Design review of the part built by this model. Coordinates are the model's own, in mm. Face numbers are marked on the shaded views. A direction names the side the tool comes from. Give positions to 0.01 mm unless a question says otherwise; leave off trailing zeros. Order: outer loops, then holes, each group sorted by start corner. A loop starts at its lowest first (then second) coordinate and runs counter-clockwise, first axis right, second up. Notation, with made-up numbers: (86.5, 16) -> (113.5, 16) arc R24 cw to (113.5, 50) -> close; hole circle Ø7 at (19.5, -29). An arc over 180 degrees is marked (long way). Use a Markdown table: item, result. Add a question column.
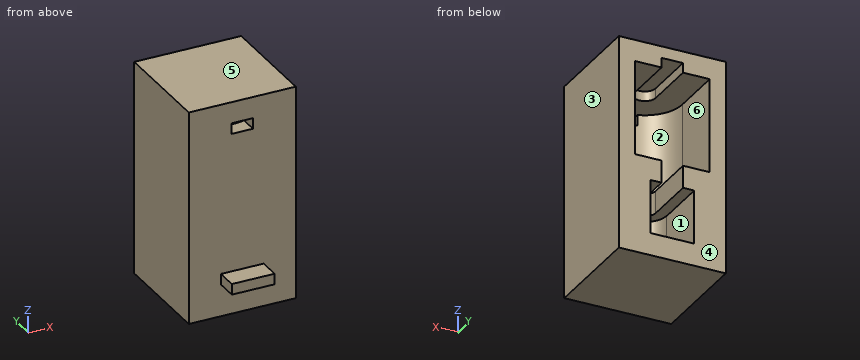
Autodesk Inventor part; units mm, degrees
ref_plane "Work Plane3" through (-14.75, 0, -89.55) normal (0, 0, -1) x (-1, 0, 0)
ref_plane "Work Plane4" through (-7.5, 0, -54) normal (0, 0, -1) x (-1, 0, 0)
ref_plane "Work Plane5" through (-14.75, 0, -64.45) normal (0, 0, -1) x (-1, 0, 0)
sketch "Sketch1" plane through (0, 0, 0) normal (0, 1, 0) x (-1, 0, 0)
  line L0 (0, 0) -> (50, 0)
  line L1 (50, 0) -> (50, -100)
  line L2 (50, -100) -> (0, -100)
  line L3 (0, -100) -> (0, 0)
  line L4 (25, 0) -> (25, -100)
  line L5 (7.5, -54) -> (7.5, -10)
  line L6 (7.5, -10) -> (42.5, -10)
  line L7 (42.5, -10) -> (42.5, -54)
  line L8 (42.5, -54) -> (7.5, -54)
  line L9 (7.5, -54) -> (42.5, -10) construction
  line L10 (7.5, -10) -> (42.5, -54) construction
  line L11 (7.5, -54) -> (51.5, -54) construction
  line L12 (14.75, -64.45) -> (14.75, -89.55)
  line L13 (14.75, -89.55) -> (35.25, -89.55)
  line L14 (35.25, -89.55) -> (35.25, -64.45)
  line L15 (35.25, -64.45) -> (14.75, -64.45)
  line L16 (14.75, -64.45) -> (35.25, -89.55) construction
  line L17 (14.75, -89.55) -> (35.25, -64.45) construction
  line L18 (14.75, -64.45) -> (39.85, -64.45) construction
  line L19 (25, -10) -> (25, -15)
  line L20 (25, -10) -> (30, -10) construction
  line L21 (20, -20) -> (30, -20)
  line L22 (30, -20) -> (30, -10)
  line L23 (30, -10) -> (20, -10)
  line L24 (20, -10) -> (20, -20)
  line L25 (20, -20) -> (30, -10) construction
  line L26 (30, -20) -> (20, -10) construction
  line L27 (20, -20) -> (30, -20) construction
  line L28 (30, -15) -> (20, -15)
  point P0 (25, -32)
  point P1 (25, -77)
  point P2 (25, -54)
  point P3 (25, -77)
  dimension "d0" = 50
  dimension "d1" = 100
  dimension "d4" = 44
  dimension "d5" = 90
  dimension "d6" = 35
  dimension "d7" = 10
  dimension "d8" = 25.1
  dimension "d9" = 90
  dimension "d10" = 20.5
  dimension "d35" = 5
  dimension "d36" = 90
  dimension "d37" = 0
extrude "Extrusion1" add sketch "Sketch1" against normal blind 50
ref_plane "Work Plane3" through (-14.75, 0, -89.55) normal (0, 0, -1) x (-1, 0, 0)
ref_plane "Work Plane4" through (-7.5, 0, -54) normal (0, 0, -1) x (-1, 0, 0)
sketch "Sketch3" plane through (-14.75, 0, -89.55) normal (0, 0, -1) x (-1, 0, 0)
  line L0 (35.25, 0) -> (-14.75, 0)
  line L1 (35.25, 0) -> (35.25, -50)
  line L2 (-14.75, -50) -> (35.25, -50)
  line L3 (-14.75, 0) -> (-14.75, -50)
  circle A0 centre (10.25, -25) radius 10.1
  line L4 (20.35, -35.1) -> (20.35, -14.9)
  line L5 (20.35, -14.9) -> (0.15, -14.9)
  line L6 (0.15, -14.9) -> (0.15, -35.1)
  line L7 (0.15, -35.1) -> (20.35, -35.1)
  line L8 (20.35, -35.1) -> (0.15, -14.9) construction
  line L9 (20.35, -14.9) -> (0.15, -35.1) construction
  line L10 (20.35, -35.1) -> (40.55, -35.1) construction
  point P0 (10.25, -35.1)
  point P1 (0.15, -25)
  point P2 (20.35, -25)
  dimension "d18" = 20.2
  dimension "d21" = 90
ref_plane "Work Plane5" through (-14.75, 0, -64.45) normal (0, 0, -1) x (-1, 0, 0)
ref_plane "Work Plane6" through (-7.5, 0, -10) normal (0, 0, -1) x (-1, 0, 0)
ref_plane "Work Plane7" through (-35.1, -35.1, -89.55) normal (0, 1, 0) x (1, 0, 0)
extrude "Extrusion5" cut sketch "Sketch1" against normal up to surface (35.1 mm away) contours L13 L12 L15 L4 | L4 L15 L14 L13
extrude "Extrusion6" add sketch "Sketch3" against normal up to surface (25.1 mm away) contours L4 L7 A0 | L7 L6 A0
sketch "Sketch4" plane through (-7.5, 0, -54) normal (0, 0, -1) x (-1, 0, 0)
  line L0 (42.5, 0) -> (-7.5, 0)
  line L1 (42.5, 0) -> (42.5, -50)
  line L2 (-7.5, -50) -> (42.5, -50)
  line L3 (-7.5, 0) -> (-7.5, -50)
  circle A0 centre (17.5, -25) radius 17.5
  line L4 (0, -42.5) -> (0, -7.5)
  line L5 (0, -7.5) -> (35, -7.5)
  line L6 (35, -7.5) -> (35, -42.5)
  line L7 (35, -42.5) -> (0, -42.5)
  line L8 (0, -42.5) -> (35, -7.5) construction
  line L9 (0, -7.5) -> (35, -42.5) construction
  line L10 (0, -42.5) -> (35, -42.5) construction
  point P0 (17.5, -42.5)
  point P1 (35, -25)
  point P2 (0, -25)
  dimension "d26" = 35
  dimension "d27" = 90
ref_plane "Work Plane8" through (-7.5, -42.5, -54) normal (0, 1, 0) x (1, 0, 0)
extrude "Extrusion7" cut sketch "Sketch1" against normal up to surface (42.5 mm away) contours L6 L22 L28 L4 | L4 L28 L24 L6 | L28 L22 L21 L4 | L4 L21 L24 L28 | L24 L21 L4 L8 L5 L6 | L6 L7 L8 L4 L21 L22
extrude "Extrusion8" add sketch "Sketch4" against normal up to surface (44 mm away) contours L6 L7 A0 | L7 L4 A0
sketch "Sketch5" plane through (-14.75, 0, -64.45) normal (0, 0, -1) x (-1, 0, 0)
  line L0 (35.25, 0) -> (-14.75, 0)
  line L1 (35.25, 0) -> (35.25, -50)
  line L2 (-14.75, -50) -> (35.25, -50)
  line L3 (-14.75, 0) -> (-14.75, -50)
  circle A0 centre (10.25, -25) radius 5
  dimension "d32" = 10
extrude "Extrusion9" cut sketch "Sketch5" against normal blind 59 contours A0
extrude "Extrusion10" cut sketch "Sketch1" against normal through all contours L6 L22 L28 L4 | L4 L28 L24 L6
ref_plane "Work Plane9" through (-25, -25, -64.45) normal (0, 1, 0) x (1, 0, 0)
sketch "Sketch6" plane through (-25, -25, -64.45) normal (0, 1, 0) x (1, 0, 0)
  line L0 (-5, 0) -> (-5, -10.45)
  line L1 (-5, 0) -> (5, 0)
  line L2 (5, -10.45) -> (-5, -10.45)
  line L3 (5, -10.45) -> (-5, -10.45)
  line L4 (-5, -10.45) -> (5, -10.45)
  line L5 (5, -10.45) -> (5, 0)
  line L6 (5, 0) -> (-5, 0)
  line L7 (-5, 0) -> (-5, -10.45)
  line L8 (-5, -59) -> (5, -59)
  line L9 (-5, -54.45) -> (-5, -59)
  line L10 (5, -54.45) -> (5, -59)
  line L11 (-5, -54.45) -> (5, -54.45)
  line L12 (5, -54.45) -> (-5, -54.45)
  line L13 (-5, -54.45) -> (-5, -59)
  line L14 (-5, -59) -> (5, -59)
  line L15 (5, -59) -> (5, -54.45)
  point P0 (25, -64.45)
extrude "Extrusion11" cut sketch "Sketch6" along normal through all
sketch "Sketch7" plane through (0, -50, 0) normal (0, -1, 0) x (1, 0, 0)
  line L0 (-50, -100) -> (0, -100)
  line L1 (-25, -100) -> (-25, -80)
  line L2 (-25, -80) -> (-35, -80)
  line L3 (-35, -80) -> (-35, -85)
  line L4 (-35, -85) -> (-25, -85)
  line L5 (-25, -85) -> (-25, -80)
  line L6 (-35, -85) -> (-15, -85)
  line L7 (-15, -85) -> (-15, -80)
  line L8 (-15, -80) -> (-35, -80)
  line L9 (-35, -80) -> (-35, -85)
  point P0 (0, 0)
  dimension "d42" = 20
  dimension "d43" = 10
  dimension "d44" = 5
  dimension "d45" = 20
extrude "Extrusion12" add sketch "Sketch7" along normal blind 10
properties part number "dcmotor_housing"
1) Add section A-A (x = -25). Give the boundary of the cut face in (y, z).
2) Add section D-D (y = -39). Give the boundary of the cut face in (x, z), then the cut area to 3 significant figures.
3) For L1, parallel to Z at x = -34.5, y = -7.5; L2, parallel to X at y = -5, z = -65; L3, parallel to Z at x = -34, y = -38, list the stretches that pass through material, from the lowest coordinate up. Write a range as [from, to].
4) Insertion check: pin 1 (10 mm diameter, centred on x = -20, z = -21.5, fed in from +Y); pin 2 (2 mm diameter, centred on x = -26.5, z = -31, fed in from -Y); pin 3 (5 mm diameter, centred on y = -8.5, z = -7.5, fed in from +X); pin 4 (3 mm diameter, centred on x = -22, y = -53, fed in from +Z). Each pin has a flat end and moves straight along its axis. Give the tip position at first contact, or say it passes through.
5) Machinability: for the marked faces 5 and 6, which of the approach directions +Z, -Z, +X, -X, +Y, -Y give a long, thin tool a straight path to every point of the face, cutting with its end or side? Answer none if there is none.
6) Add section B-B (y = -9.5). Give the boundary of the cut face in (x, z).
7) Add section C-C (z = -49). Give the boundary of the cut face in (x, y).
8) The part is to be moulded in two halves that separate along X. For the marked faces 1, 2, 3 and 4, say which applies: +X half, -X half, draft (parallel to the pull), parting line (faces both ways), or undercut.
Worked answers:
| question | item | result |
|---|---|---|
| 1 | outline | (-60, -85) -> (-50, -85) -> (-50, -100) -> (0, -100) -> (0, -89.55) -> (-35.1, -89.55) -> (-35.1, -64.45) -> (-30, -64.45) -> (-30, -54) -> (-42.5, -54) -> (-42.5, -15) -> (-50, -15) -> (-50, -80) -> (-60, -80) -> close; (-50, -10) -> (-30, -10) -> (-30, -5.45) -> (0, -5.45) -> (0, 0) -> (-50, 0) -> close |
| 2 | outline | (-50, -100) -> (0, -100) -> (0, 0) -> (-50, 0) -> close; hole (-35.5, -54) -> (-14.5, -54) -> (-14.5, -10) -> (-35.5, -10) -> close |
| 2 | area | 4,080 mm^2 |
| 3 | L1 | [-100, -89.55], [-64.45, -54], [-10, 0] |
| 3 | L2 | [-50, -35.25], [-14.75, 0] |
| 3 | L3 | [-100, -54], [-10, 0] |
| 4 | pin 1 | y = -39.36 |
| 4 | pin 2 | y = -50 |
| 4 | pin 3 | x = 0 |
| 4 | pin 4 | z = -80 |
| 5 | face 5 | +Z, +X, -X, +Y, -Y |
| 5 | face 6 | +Y |
| 6 | outline | (-50, -100) -> (0, -100) -> (0, 0) -> (-50, 0) -> close; hole (-42.5, -54) -> (-30, -54) -> (-30, -64.45) -> (-35.25, -64.45) -> (-35.25, -89.55) -> (-14.75, -89.55) -> (-14.75, -64.45) -> (-20, -64.45) -> (-20, -54) -> (-7.5, -54) -> (-7.5, -10) -> (-20, -10) -> (-20, -5.45) -> (-30, -5.45) -> (-30, -10) -> (-42.5, -10) -> close |
| 7 | outline | (-50, -50) -> (0, -50) -> (0, 0) -> (-7.5, 0) -> (-7.5, -25) arc R17.5 cw to (-42.5, -25) -> (-42.5, 0) -> (-50, 0) -> close |
| 8 | face 1 | undercut |
| 8 | face 2 | undercut |
| 8 | face 3 | +X half |
| 8 | face 4 | draft |
